```python
from build123d import *

# Parameters (mm, degrees)
TROU_TARAUD_M61_D     = 5
TROU_TARAUD_M61_DEPTH = 20
TROU_TARAUD_M61_TIP   = 1.502151548
EXTRUSION1_DEPTH      = 22.650635095
EXTRUSION1_DEPTH_BACK = 22.650635095
ESQUISSE5_W           = 11.874342088
ESQUISSE5_H           = 3.786271938


with BuildPart() as part:
    # Esquisse1 → Révolution1 (revolve)
    with BuildSketch(Plane.XY):
        with BuildLine():
            Line((0, -12.5), (0, 12.5))
            ThreePointArc((0, 12.5), (12.5, 0), (0, -12.5))
        make_face()
    revolve(axis=Axis((0, 81.368836261, 0), (0, -1, 0)))

    # Trou taraudé M61
    with Locations(Plane(origin=(0, 12.5, 0), x_dir=(-1, 0, 0), z_dir=(0, 1, 0))):
        with Locations((0, 0)):
            Hole(TROU_TARAUD_M61_D / 2, depth=TROU_TARAUD_M61_DEPTH)
            with Locations((0, 0, -(TROU_TARAUD_M61_DEPTH + TROU_TARAUD_M61_TIP / 2))):  # 118° drill point
                Cone(0, TROU_TARAUD_M61_D / 2, TROU_TARAUD_M61_TIP, mode=Mode.SUBTRACT)

    # Esquisse5 → Extrusion1 (cut, two sides: drawn at the far end of the back side and taken through both)
    with BuildSketch(Plane.XY.offset(-EXTRUSION1_DEPTH_BACK)):
        with Locations((0, 12.893135969)):
            Rectangle(ESQUISSE5_W, ESQUISSE5_H)
    extrude(amount=EXTRUSION1_DEPTH + EXTRUSION1_DEPTH_BACK, mode=Mode.SUBTRACT)


solid = part.part
```
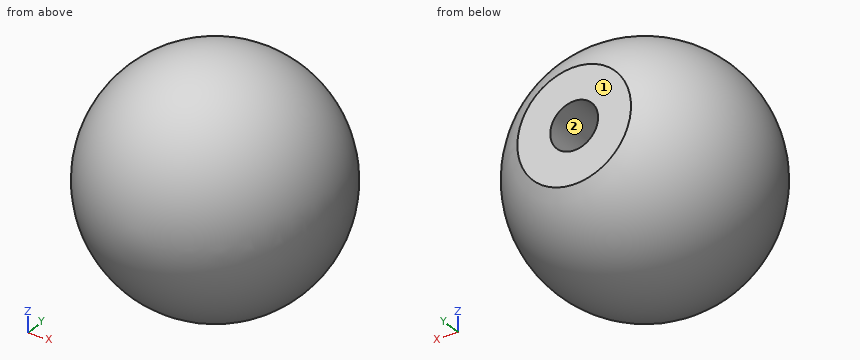
Design review of the part built by this model. Coordinates are the model's own, in mm. Face numbers are marked on the shaded views. Give positions to 0.01 mm unless a question says otherwise; leave off trailing zeros. Loops run counter-clockwise (first coordinate to the right, second up) from the corner with the lowest first, then second, coordinate; pieces in that order, holes last. Notation, with made-up numbers: M 53,13 L 103,13 A18 cw 103,24 Z; hole C -17.75,68 d1. An arc over 180 degrees is marked long. Return JSON: item names as keys, results as strings. Group by question number.
Item 1: Mouldability with a two-part tool opening along Z and no side actions: class the marked faces 1 and 2 as released by +Z, released by -Z, zero draft, split by the parting line, or undercut.
Item 2: We need section D-D (y = -0.75). Give the boundary of the cut face in (x, z).
Item 3: We need section C-C (x = -4.5). Give the boundary of the cut face in (y, z).
Item 4: Insertion check: pin 1 Ø3 at (y, z) = (7, -5.5) entering from -X; pin 2 Ø1 at (x, y) = (0, -3.5) entering from +Z; pin 3 Ø10 at (x, y) = (-1, 6) entering from +Z. Each pin has a flat end and moves straight along its axis. Give the tip position at first contact, or say it passes through.
Item 5: We need section A-A (y = 8.75). Give the boundary of the cut face in (x, z), and give its area (3 significant figures).
Item 6: We need section B-B (z = 7.75). Give the boundary of the cut face in (x, y).
Item 7: For probe 1 along Z at (x, y) = (0, 0.25); probe 2 along X at (y, z) = (5.5, 0); probe 3 along Z at (x, y) = (0, 7), list the stretches that pass through material, from the lowest coordinate up.
Output:
{
 "1": {"face 1": "zero draft", "face 2": "undercut"},
 "2": {"outline": "C 0,0 d24.95; hole C 0,0 d5"},
 "3": {"outline": "M 11,-3.87 L 11,3.87 A11.66 ccw long Z"},
 "4": {"pin 1": "stops at x = -10.07", "pin 2": "stops at z = 12.13", "pin 3": "stops at z = 12.45"},
 "5": {"outline": "C 0,0 d17.85; hole C 0,0 d5", "area": "231 mm^2"},
 "6": {"outline": "C 0,0 d19.62"},
 "7": {"probe 1": "z = -12.5 to -2.5, 2.5 to 12.5", "probe 2": "x = -11.22 to -2.5, 2.5 to 11.22", "probe 3": "z = -10.36 to -2.5, 2.5 to 10.36"}
}
